Drawing for the job (mm, zero at the part's lowest x, y, z). A direction names the side the tool comes from. Coordinates: 2 decimals unless noted, no trailing zeros. Loops run counter-clockwise (first coordinate to the right, second up) from the corner with the lowest first, then second, coordinate; pieces in that order, holes last. Notation, with made-up numbers: (39, 51.25) - (92, 51.25) arc R16 ccw to (92, 63.25) - close; hole circle Ø5 at (88.25, 74). An arc over 180 degrees is marked (long way). One line per item, written item: value.
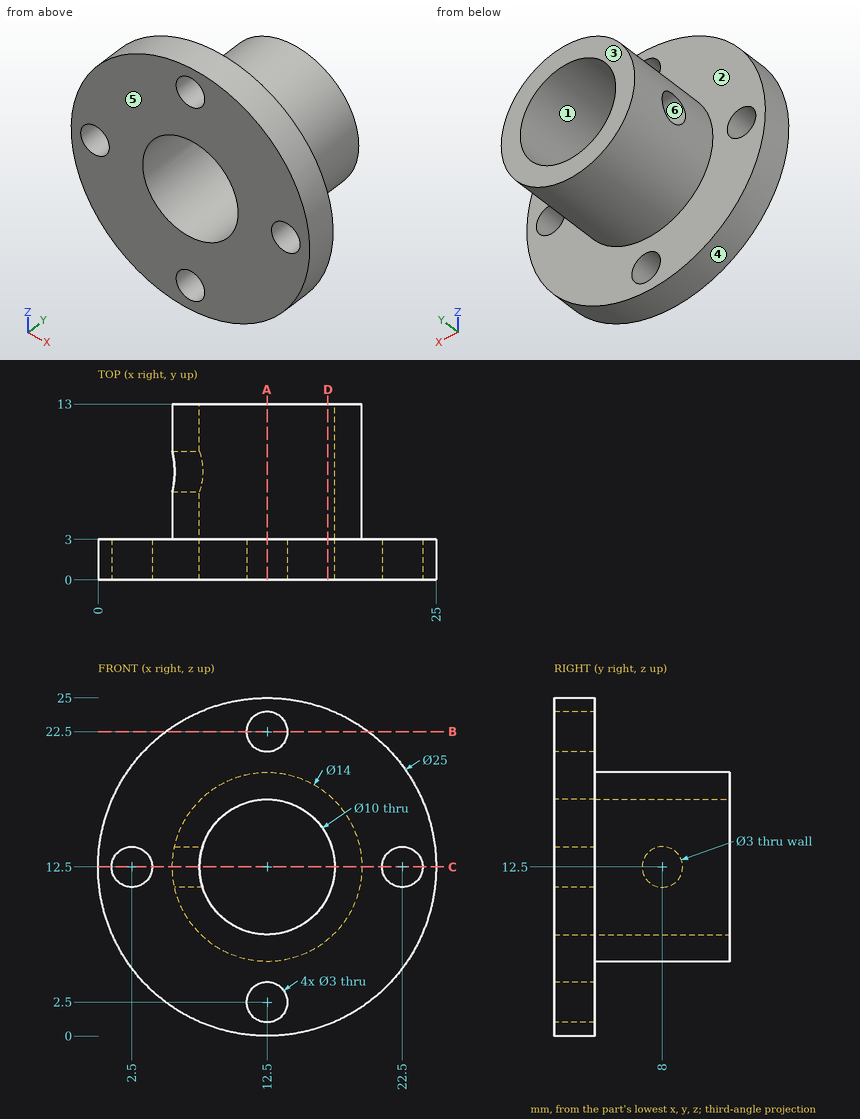
Item 1: Probe probe 1 along X at (y, z) = (5, 12.5); probe 2 along Y at (x, z) = (16.5, 1.75). List the from-to ranges inside material, lowest first. Write a range as from..to.
Check result:
probe 1: x = 5.5..7.5, 17.5..19.5
probe 2: y = 0..3
Item 2: Tool access for the marked faces 1 and 2: list every direction of +Z, -Z, +X, -X, +Y, -Y with a clear straight run to the whole face (end or side of a thin tool).
Check result:
face 1: +Y, -Y
face 2: +Y
Item 3: Drop flat-ended pins along their axis: P1, Ø2.5, axis at x = 12.5, z = 2.5, coming from the -Y side; P2, Ø2, axis at y = 5.5, z = 9, coming from the +X side; P3, Ø4, axis at x = 10.5, y = 6.5, coming from the -Z side; P4, Ø1, axis at x = 18.5, y = 7.5, coming from the +Z side. Give the stop position or say it passes through.
Check result:
P1: passes through
P2: stops at x = 19.04
P3: stops at z = 5.5
P4: stops at z = 16.83
Item 4: Pull direction Y, two halves, no side cores. Call the marked faces 3, 4, 5 and 6: released by +Y, released by -Y, zero draft, split by the parting line, or undercut.
Check result:
face 3: released by +Y
face 4: zero draft
face 5: released by -Y
face 6: undercut
Item 5: Cut at B-B, the plane z = 22.5. Write the cut outline in (x, y).
Check result:
outline: (5, 0) - (11, 0) - (11, 3) - (5, 3) - close; (14, 0) - (20, 0) - (20, 3) - (14, 3) - close
Item 6: Cut at C-C, the plane z = 12.5. Write the cut outline in (x, y), then the cut area to 3 significant figures.
Check result:
outline: (0, 0) - (1, 0) - (1, 3) - (0, 3) - close; (4, 0) - (7.5, 0) - (7.5, 6.5) - (5.5, 6.5) - (5.5, 3) - (4, 3) - close; (5.5, 9.5) - (7.5, 9.5) - (7.5, 13) - (5.5, 13) - close; (17.5, 0) - (21, 0) - (21, 3) - (19.5, 3) - (19.5, 13) - (17.5, 13) - close; (24, 0) - (25, 0) - (25, 3) - (24, 3) - close
area: 61.0 mm^2
Item 7: Cut at D-D, the plane x = 17. Write the cut outline in (y, z), then the cut area to 3 significant figures.
Check result:
outline: (0, 0.84) - (3, 0.84) - (3, 7.14) - (13, 7.14) - (13, 10.32) - (0, 10.32) - close; (0, 14.68) - (13, 14.68) - (13, 17.86) - (3, 17.86) - (3, 24.16) - (0, 24.16) - close
area: 121 mm^2
Item 8: Cut at A-A, the plane x = 12.5. Write the cut outline in (y, z).
Check result:
outline: (0, 0) - (3, 0) - (3, 1) - (0, 1) - close; (0, 4) - (3, 4) - (3, 5.5) - (13, 5.5) - (13, 7.5) - (0, 7.5) - close; (0, 17.5) - (13, 17.5) - (13, 19.5) - (3, 19.5) - (3, 21) - (0, 21) - close; (0, 24) - (3, 24) - (3, 25) - (0, 25) - close
